Input: part model. Units: mm. Frame: model coordinates. Coordinates: 2 decimals unless noted, no trailing zeros.
Autodesk Inventor part; units mm, degrees
ref_plane "YZ Plane" through (0, 0, 0) normal (1, 0, 0) x (0, 1, 0)
ref_plane "XZ Plane" through (0, 0, 0) normal (0, 1, 0) x (-1, 0, 0)
ref_plane "XY Plane" through (0, 0, 0) normal (0, 0, 1) x (1, 0, 0)
sketch "Sketch1" plane through (0, 0, 0) normal (0, 1, 0) x (-1, 0, 0)
  line L0 (31.64, 0) -> (-31.64, 0) construction
  line L1 (0, -27.44) -> (0, 27.44) construction
  line L2 (-22.6, 19.6) -> (22.6, 19.6)
  line L3 (22.6, 19.6) -> (22.6, -19.6)
  line L4 (22.6, -19.6) -> (-22.6, -19.6)
  line L5 (-22.6, -19.6) -> (-22.6, 19.6)
  line L6 (-22.6, 0) -> (22.6, 0) construction
  point P0 (0, 0)
  dimension "d0" = 45.2
  dimension "d1" = 39.2
extrude "Extrusion1" add sketch "Sketch1" along normal blind 4
fillet "Fillet1" radius 5.2 4 edges at (-22.6, 2, 19.6) (22.6, 2, 19.6) (22.6, 2, -19.6) (-22.6, 2, -19.6)
properties part number "plexiglas_4mm" material "Glass"
Item 1: Line query: L1, parallel to Z at x = -20, y = 1.35; L2, parallel to Z at x = -19, y = 3. Output: solid intervals per line, ascending.
Result:
L1: z = -18.9 to 18.9
L2: z = -19.35 to 19.35
Item 2: Mould query, pull axis Z, two halves, no side actions, for faces 1 (the face through (-21.036, 2.028, -18.117)), 2 (the face through (21.036, 2.028, 18.117)), 3 (the face through (0, 0, 0)). Classes: +Z half, -Z half, draft (parallel to the pull), parting line (faces both ways), or undercut.
Result:
face 1: -Z half
face 2: +Z half
face 3: draft
Item 3: Contact query for a flat-ended pin moving along its axis: P1, Ø3, axis at x = 7.5, z = -5.5, coming from the -Y side. Output: stop coordinate, or through.
Result:
P1: stops at y = 0
